Autodesk Inventor part; units mm, degrees
ref_plane "YZ Plane" through (0, 0, 0) normal (1, 0, 0) x (0, 1, 0)
ref_plane "XZ Plane" through (0, 0, 0) normal (0, 1, 0) x (-1, 0, 0)
ref_plane "XY Plane" through (0, 0, 0) normal (0, 0, 1) x (1, 0, 0)
sketch "Sketch1" plane through (0, 0, 0) normal (0, 1, 0) x (-1, 0, 0)
  line L0 (8, 0) -> (8, 8)
  line L1 (8, 8) -> (0, 8)
  line L2 (0, 8) -> (0, 0)
  line L3 (0, 0) -> (8, 0)
  line L4 (8, 0) -> (8, 8)
  line L5 (49.4, -65) -> (41.4, -65)
  line L6 (49.4, -65) -> (41.4, -65)
  line L7 (41.4, -65) -> (41.4, -73)
  line L8 (41.4, -73) -> (49.4, -73)
  line L9 (49.4, -73) -> (49.4, -65)
  line L10 (80, -35.15) -> (80, -43.15)
  line L11 (88, -35.15) -> (80, -35.15)
  line L12 (80, -35.15) -> (80, -43.15)
  line L13 (80, -43.15) -> (88, -43.15)
  line L14 (88, -43.15) -> (88, -35.15)
  line L15 (-22.4, -65) -> (-14.4, -65)
  line L16 (-22.4, -73) -> (-22.4, -65)
  line L17 (-14.4, -65) -> (-22.4, -65)
  line L18 (-22.4, -65) -> (-22.4, -73)
  line L19 (-22.4, -73) -> (-14.4, -73)
  line L20 (-14.4, -73) -> (-14.4, -65)
  line L21 (-72, -43.15) -> (-72, -35.15)
  line L22 (-80, -43.15) -> (-72, -43.15)
  line L23 (-72, -35.15) -> (-80, -35.15)
  line L24 (-80, -35.15) -> (-80, -43.15)
  line L25 (-80, -43.15) -> (-72, -43.15)
  line L26 (-72, -43.15) -> (-72, -35.15)
  circle A0 centre (-76, -39.15) radius 1.6
  circle A1 centre (-18.4, -69) radius 1.6
  circle A2 centre (45.4, -69) radius 1.6
  circle A3 centre (84, -39.15) radius 1.6
  circle A4 centre (4, 4) radius 1.6
  line L27 (0, 0) -> (8, 0)
  line L28 (41.4, -65) -> (41.4, -73)
  line L29 (41.4, -73) -> (-14.4, -73)
  line L30 (-80, -43.15) -> (-22.4, -73)
  line L31 (88, -43.15) -> (49.4, -73)
  line L32 (0, 8) -> (0, 0)
  line L33 (0, 8) -> (-72, -35.15)
  line L34 (8, 8) -> (80, -35.15)
  line L35 (80, -39.15) -> (8, 4)
  line L36 (0, 4) -> (-72, -39.15)
  line L37 (-22.4, -69) -> (-72.2814, -43.15)
  line L38 (80, -43.15) -> (49.4, -69)
  line L39 (49.4, -73) -> (49.4, -65)
  line L40 (41.4, -69) -> (-14.4, -69)
  line L41 (-14.4, -65) -> (-14.4, -73)
  line L42 (4, 0) -> (45.4, -65)
  line L43 (8, 0) -> (49.4, -65)
  line L44 (0, 0) -> (-22.4, -65)
  line L45 (-18.4, -65) -> (4, 0)
  point P0 (-14.4, -69)
  dimension "d0" = 3.2
extrude "Extrusion1" add sketch "Sketch1" along normal blind 2 contours L3 L2 L1 L0 | L43 L5 L42 L3 | L0 L34 L10 L35 | L45 L15 L44 L3 | L9 L8 L7 L5 | L10 L11 L14 L13 | L15 L20 L19 L16 | L38 L13 L31 L9 | L2 L36 L21 L33 | L21 L22 L24 L23 | L16 L30 L22 L37 | L7 L29 L20 L40
properties part number "ScrewHoleGuide"
Geometry: final body of the model. Coordinates: model frame, mm. A direction names the side the tool comes from. Round coordinates to 2 decimals unless told otherwise and drop trailing zeros. Loops run counter-clockwise (first coordinate to the right, second up) from the corner with the lowest first, then second, coordinate; pieces in that order, holes last.
Item 1: Section B-B, the plane x = 7. Output: boundary loops of the cut face in (y, z), plus the area to 3 significant figures.
Checked values:
outline: (0, -73) - (2, -73) - (2, -69) - (0, -69) - close; (0, -31.92) - (2, -31.92) - (2, -20.31) - (0, -20.31) - close; (0, -0.2) - (2, -0.2) - (2, 3.8) - (0, 3.8) - close
area: 39.2 mm2
Item 2: Mould query, pull axis Z, two halves, no side actions, for faces 1 (the flat face through (9, 2, -35)), 2 (the flat face through (-28.41, 0.986, -32.045)), 3 (the flat face through (51.603, 0.986, -57.866)). Classes: released by +Z, released by -Z, zero draft, split by the parting line, or undercut.
Checked values:
face 1: zero draft
face 2: undercut
face 3: released by -Z
Item 3: Line query: L1, parallel to X at y = 1.35, z = -38.5; L2, parallel to X at y = 1.5, z = -29.5; L3, parallel to X at y = 1.55, z = -30. Output: solid intervals per line, ascending.
Checked values:
L1: x = -88 to -85.46, -82.54 to -78.92, -32.52 to -28.52, 9.27 to 13.27, 70.92 to 74.54, 77.46 to 80
L2: x = -70.57 to -63.9, -26.79 to -22.79, 6.17 to 10.17, 55.9 to 62.57
L3: x = -71.41 to -64.73, -27.11 to -23.11, 6.34 to 10.34, 56.73 to 63.41
Item 4: Reachability of faces 4 (the flat face through (9, 0, -35)), 5 (the flat face through (46.992, 0.986, -56.256)) from +Z, -Z, +X, -X, +Y, -Y: full face, straight path, thin tool, end or side. Return the list, or none.
Checked values:
face 4: +Z, -Z, +X, -X, -Y
face 5: +Y, -Y
Item 5: Section A-A, the plane z = -49.5. Output: boundary loops of the cut face in (x, y).
Checked values:
outline: (-79.79, 0) - (-72.48, 0) - (-72.48, 2) - (-79.79, 2) - close; (-39.53, 0) - (-35.53, 0) - (-35.53, 2) - (-39.53, 2) - close; (13.06, 0) - (17.06, 0) - (17.06, 2) - (13.06, 2) - close; (60.03, 0) - (67.75, 0) - (67.75, 2) - (60.03, 2) - close
Item 6: Section D-D, the plane y = 0.6. State how many separate pieces and enclosed holes the cut face has, plus the area to 3 significant figures.
Checked values:
separate pieces: 1
enclosed holes: 8
area: 1,990 mm2
Item 7: Section C-C, the plane x = 76. Output: boundary loops of the cut face in (y, z).
Checked values:
outline: (0, -45.22) - (2, -45.22) - (2, -40.75) - (0, -40.75) - close; (0, -37.55) - (2, -37.55) - (2, -35.15) - (0, -35.15) - close
Item 8: Contact query for flat-ended pins moving along their axis: P1, Ø0.6, axis at x = -42.5, y = 1, coming from the +Z side; P2, Ø1.9, axis at x = -45.4, z = -69, coming from the +Y side; P3, Ø1, axis at y = 1.5, z = -66.5, coming from the -X side; P4, Ø0.6, axis at y = 1, z = -67.5, coming from the +X side. Output: stop coordinate, or through.
Checked values:
P1: stops at z = -12.5
P2: passes through
P3: stops at x = -58.45
P4: stops at x = 33.59
